from build123d import *

# Parameters (mm, degrees)
SKETCH2_R               = 10
SKETCH2_R_2             = 3
BOSS_EXTRUDE1_DEPTH     = 4
CUT_EXTRUDE3_DEPTH      = 128.285567155
CUT_EXTRUDE3_DEPTH_BACK = 128.285567155


with BuildPart() as part:
    # Sketch2 → Boss-Extrude1 (new body)
    with BuildSketch(Plane(origin=(0, 0, 0), x_dir=(0, 0, -1), z_dir=(1, 0, 0))):
        with BuildLine():
            Line((119, 9), (119, 44.995728753))
            Line((119, 44.995728753), (94, 44.995728753))
            Line((94, 44.995728753), (94, 24.715728753))
            ThreePointArc((94, 24.715728753), (89.39696962, 13.60303038), (78.284271247, 9))
            ThreePointArc((78.284271247, 9), (71.617604581, 10.143819168), (65.713484026, 13.444444444))
            ThreePointArc((65.713484026, 13.444444444), (50, 19), (34.286515974, 13.444444444))
            ThreePointArc((34.286515974, 13.444444444), (28.382395419, 10.143819168), (21.715728753, 9))
            Line((21.715728753, 9), (-20, 9))
            Line((-20, 9), (-27.928932188, 1.071067812))
            Line((-27.928932188, 1.071067812), (-30.757359313, 3.899494937))
            Line((-30.757359313, 3.899494937), (-44.899494937, -10.242640687))
            Line((-44.899494937, -10.242640687), (-42.071067812, -13.071067812))
            Line((-42.071067812, -13.071067812), (-50, -21))
            Line((-50, -21), (18.196601125, -21))
            Line((18.196601125, -21), (30, -21))
            Line((30, -21), (90, -41))
            Line((90, -41), (90, -21))
            Line((90, -21), (94, -21))
            Line((94, -21), (94, -41))
            Line((94, -41), (119, 9))
        make_face()
        with Locations((50, -6)):
            Circle(SKETCH2_R, mode=Mode.SUBTRACT)
        with Locations((106.5, -6)):
            Circle(SKETCH2_R_2, mode=Mode.SUBTRACT)
        with Locations((106.5, 4)):
            Circle(SKETCH2_R_2, mode=Mode.SUBTRACT)
        with Locations((113, 9)):
            Circle(SKETCH2_R_2, mode=Mode.SUBTRACT)
        with Locations((106.5, 14)):
            Circle(SKETCH2_R_2, mode=Mode.SUBTRACT)
        with Locations((113, 19)):
            Circle(SKETCH2_R_2, mode=Mode.SUBTRACT)
        with Locations((106.5, 24)):
            Circle(SKETCH2_R_2, mode=Mode.SUBTRACT)
        with Locations((113, 29)):
            Circle(SKETCH2_R_2, mode=Mode.SUBTRACT)
        with Locations((113, 39)):
            Circle(SKETCH2_R_2, mode=Mode.SUBTRACT)
        with Locations((106.5, 34)):
            Circle(SKETCH2_R_2, mode=Mode.SUBTRACT)
        with Locations((100, 39)):
            Circle(SKETCH2_R_2, mode=Mode.SUBTRACT)
        with Locations((100, 29)):
            Circle(SKETCH2_R_2, mode=Mode.SUBTRACT)
        with Locations((100, 19)):
            Circle(SKETCH2_R_2, mode=Mode.SUBTRACT)
        with Locations((100, 9)):
            Circle(SKETCH2_R_2, mode=Mode.SUBTRACT)
        with Locations((100, -1)):
            Circle(SKETCH2_R_2, mode=Mode.SUBTRACT)
        with Locations((100, -11)):
            Circle(SKETCH2_R_2, mode=Mode.SUBTRACT)
        with Locations((84, 4)):
            Circle(SKETCH2_R_2, mode=Mode.SUBTRACT)
        with Locations((71, 4)):
            Circle(SKETCH2_R_2, mode=Mode.SUBTRACT)
        with Locations((77.5, -1)):
            Circle(SKETCH2_R_2, mode=Mode.SUBTRACT)
        with Locations((84, -6)):
            Circle(SKETCH2_R_2, mode=Mode.SUBTRACT)
        with Locations((84, -16)):
            Circle(SKETCH2_R_2, mode=Mode.SUBTRACT)
        with Locations((77.5, -11)):
            Circle(SKETCH2_R_2, mode=Mode.SUBTRACT)
        with Locations((71, -6)):
            Circle(SKETCH2_R_2, mode=Mode.SUBTRACT)
        with Locations((71, -16)):
            Circle(SKETCH2_R_2, mode=Mode.SUBTRACT)
        with Locations((84, -26)):
            Circle(SKETCH2_R_2, mode=Mode.SUBTRACT)
        with Locations((77.5, -21)):
            Circle(SKETCH2_R_2, mode=Mode.SUBTRACT)
        with BuildLine():
            Line((20, 0), (-20, 0))
            ThreePointArc((-20, 0), (-26, -6), (-20, -12))
            Line((-20, -12), (20, -12))
            ThreePointArc((20, -12), (26, -6), (20, 0))
        make_face(mode=Mode.SUBTRACT)
    extrude(amount=BOSS_EXTRUDE1_DEPTH)

    # Sketch3 → Cut-Extrude3 (cut, two sides: drawn at the far end of the back side and taken through both)
    with BuildSketch(Plane(origin=(0, 0, 0), x_dir=(0, 0, -1), z_dir=(1, 0, 0)).offset(-CUT_EXTRUDE3_DEPTH_BACK)):
        Polygon((94, -21), (94, 9), (78.284271247, 9), (78.284271247, 52.431858837), (131.189267146, 52.431858837), (131.189267146, -47.367568871), (90.840116585, -47.367568871), align=None)
    extrude(amount=CUT_EXTRUDE3_DEPTH + CUT_EXTRUDE3_DEPTH_BACK, mode=Mode.SUBTRACT)


solid = part.part
Work out the finished part from the listing and answer in its coordinate system (mm). A direction names the side the tool comes from. Coordinates: 2 decimals unless noted, no trailing zeros. Loops run counter-clockwise (first coordinate to the right, second up) from the corner with the lowest first, then second, coordinate; pieces in that order, holes last. Notation, with made-up numbers: M -22.5,84 L 14.5,84 A8 cw 14.5,96 Z; hole C 8.5,53 d3. An arc over 180 degrees is marked long. Answer in a Markdown table with one row per item. Add a question column.
1. A tool of negligible diameter and unlimited length cuts with its end or side. For faces 1 (the flat face through (2, 0, 0)), 2 (the flat face through (2, 9, -1)), 3 (the flat face through (1.972, 2.465, 29.323)), from which of +Z, -Z, +X, -X, +Y, -Y can it reach the whole face along a straight path? Write none if from no direction.
2. Consider L1, parallel to Y at x = 3.8, z = 0.5; L2, parallel to Z at x = 2.7, y = 2.5; L3, parallel to Y at x = 1.85, z = -71. Determine where each line is inside the solid, lowest interval first.
3. Find section B-B, the plane x = 1.75. State how many separate pieces and enclosed holes the cut face has, then the cut area to 3 significant figures.
4. Find section A-A, the plane y = -26. Write down the section's boundary in (x, z).
5. The mould has two halves that part along Z. Classify faces 4 (the cylindrical face through (2, -26, -81)), 5 (the flat face through (2, -21, -92)), 6 (the cylindrical face through (2, -17.8, -81.6)), 7 (the flat face through (2, -31, -90)): pulls with the +Z half, pulls with the -Z half, needs draft (parallel to the pull), parting line crosses it, or undercut.
6. Find section C-C, the plane z = -50. Write down the section's boundary in (x, y).
7. Find section D-D, the plane y = -6. Write down the section's boundary in (x, z).
8. Flat-ended cylindrical pins translate along their axes: P1, Ø2, axis at x = 2.5, z = 20, coming from the -Y side; P2, Ø1.5, axis at x = 2, y = 4, coming from the +Z side; P3, Ø1.2, axis at x = 1, y = -30, coming from the -Z side. Find the tip coordinate at first contact, or state that the pin passes through.
Reported:
| question | item | result |
|---|---|---|
| 1 | face 1 | +X, -X |
| 1 | face 2 | +Z, +X, -X, +Y |
| 1 | face 3 | +X, -X, +Y |
| 2 | L1 | y = -21 to -12, 0 to 9 |
| 2 | L2 | z = -94 to -86.6, -81.4 to -73.6, -68.4 to -55.27, -44.73 to 26.5, 29.36 to 32.16 |
| 2 | L3 | y = -34.67 to -19, -13 to -9, -3 to 1, 7 to 10.37 |
| 3 | separate pieces | 1 |
| 3 | enclosed holes | 12 |
| 3 | area | 3,650 mm^2 |
| 4 | outline | M 0,-90 L 4,-90 L 4,-87 L 0,-87 Z; M 0,-81 L 4,-81 L 4,-45 L 0,-45 Z |
| 5 | face 4 | undercut |
| 5 | face 5 | needs draft |
| 5 | face 6 | undercut |
| 5 | face 7 | pulls with the -Z half |
| 6 | outline | M 0,-27.67 L 4,-27.67 L 4,-16 L 0,-16 Z; M 0,4 L 4,4 L 4,19 L 0,19 Z |
| 7 | outline | M 0,-94 L 4,-94 L 4,-87 L 0,-87 Z; M 0,-81 L 4,-81 L 4,-74 L 0,-74 Z; M 0,-68 L 4,-68 L 4,-60 L 0,-60 Z; M 0,-40 L 4,-40 L 4,-26 L 0,-26 Z; M 0,26 L 4,26 L 4,40.66 L 0,40.66 Z |
| 8 | P1 | stops at y = -21 |
| 8 | P2 | stops at z = 31.41 |
| 8 | P3 | stops at z = -90 |
